```python
from build123d import *

# Parameters (mm, degrees)
CROQUIS1_W                   = 30
CROQUIS1_H                   = 10
CROQUIS1_R                   = 1.6
SALIENTE_EXTRUIR1_DEPTH      = 5
CROQUIS2_R                   = 2.8
CORTAR_EXTRUIR1_DEPTH        = 3
SALIENTE_EXTRUIR2_DEPTH      = 10
SALIENTE_EXTRUIR2_DEPTH_BACK = 30
CROQUIS3_W                   = 3
CROQUIS3_H                   = 40
CROQUIS4_W                   = 10
CROQUIS4_H                   = 5
SALIENTE_EXTRUIR3_DEPTH      = 10
SALIENTE_EXTRUIR4_DEPTH      = 10
REDONDEO1_R                  = 5


with BuildPart() as part:
    # Croquis1 → Saliente-Extruir1 (new body)
    with BuildSketch(Plane(origin=(0, 0, 0), x_dir=(1, 0, 0), z_dir=(0, 1, 0))):
        with Locations((15, 5)):
            Rectangle(CROQUIS1_W, CROQUIS1_H)
        with Locations(Location((5, 5, 0), (0, 0, 270))):
            Circle(CROQUIS1_R, mode=Mode.SUBTRACT)
        with Locations(Location((25, 5, 0), (0, 0, 270))):
            Circle(CROQUIS1_R, mode=Mode.SUBTRACT)
    extrude(amount=SALIENTE_EXTRUIR1_DEPTH)

    # Croquis2 → Cortar-Extruir1 (cut)
    with BuildSketch(Plane(origin=(0, 5, 0), x_dir=(1, 0, 0), z_dir=(0, 1, 0))):
        with Locations(Location((5, 5, 0), (0, 0, 270))):
            Circle(CROQUIS2_R)
        with Locations(Location((25, 5, 0), (0, 0, 270))):
            Circle(CROQUIS2_R)
    extrude(amount=-CORTAR_EXTRUIR1_DEPTH, mode=Mode.SUBTRACT)

    # Croquis3 → Saliente-Extruir2 (add, two sides: drawn at the far end of the back side and taken through both)
    with BuildSketch(Plane.ZY.offset(-SALIENTE_EXTRUIR2_DEPTH_BACK)):
        with Locations((-11.5, 20)):
            Rectangle(CROQUIS3_W, CROQUIS3_H)
    extrude(amount=SALIENTE_EXTRUIR2_DEPTH + SALIENTE_EXTRUIR2_DEPTH_BACK)

    # Croquis4 → Saliente-Extruir3 (add)
    with BuildSketch(Plane.ZY):
        with Locations((-5, 2.5)):
            Rectangle(CROQUIS4_W, CROQUIS4_H)
    extrude(amount=SALIENTE_EXTRUIR3_DEPTH)

    # Croquis5 → Saliente-Extruir4 (add)
    with BuildSketch(Plane(origin=(30, 0, 0), x_dir=(0, 0, -1), z_dir=(1, 0, 0))):
        Polygon((0, 0), (13, 0), (13, 40), (10, 40), (10, 5), (0, 5), align=None)
    extrude(amount=SALIENTE_EXTRUIR4_DEPTH)

    # Redondeo1
    # the kernel refuses this fillet: 5 mm, written as the material it adds along each edge
    with BuildSketch(Plane(origin=(40, 5, -10), x_dir=(0, 1, 0), z_dir=(-1, 0, 0))) as redondeo1_piece_1_section:
        with BuildLine():
            CenterArc((REDONDEO1_R, -REDONDEO1_R), REDONDEO1_R, 90, 90)
            Line((0, -REDONDEO1_R), (0, 0))
            Line((0, 0), (REDONDEO1_R, 0))
        make_face()
    redondeo1_piece_1 = extrude(amount=50, mode=Mode.PRIVATE)
    redondeo1_piece_1 = redondeo1_piece_1 - Plane(origin=(5, 6.156265405, -5), x_dir=(0, 0, 1), z_dir=(0, 1, 0)) * Cylinder(2.8, 120, mode=Mode.PRIVATE)
    redondeo1_piece_1 = redondeo1_piece_1 - Plane(origin=(25, 6.156265405, -5), x_dir=(0, 0, 1), z_dir=(0, 1, 0)) * Cylinder(2.8, 120, mode=Mode.PRIVATE)
    add(redondeo1_piece_1)


solid = part.part
```
Geometry: final body of the model. Coordinates: model frame, mm. A direction names the side the tool comes from. Coordinates: 2 decimals unless noted, no trailing zeros. Order: outer loops, then holes, each group sorted by start corner. A loop starts at its lowest first (then second) coordinate and runs counter-clockwise, first axis right, second up. Notation, with made-up numbers: (64.25, 8) - (101.25, 8) arc R28 cw to (101.25, 42) - close; hole circle Ø10 at (13.5, 86.25). An arc over 180 degrees is marked (long way). Return JSON: item names as keys, results as strings. Group by question number.
1. Set-up query: faces 1 (the face through (-10, 14.2, -10.4)), 2 (the face through (15, 5, -3)), 3 (the face through (5.1, 3.5, -7.8)). Return all of +Z, -Z, +X, -X, +Y, -Y with unobstructed straight access to the full face (end or side cutting, diameter ignored); none if empty.
2. Cut plane B-B (y = 3.5). Output: boundary loops of the cut face in (x, z).
3. Cut plane C-C (x = 12). Output: boundary loops of the cut face in (y, z).
4. Cut plane A-A (x = 5). Output: boundary loops of the cut face in (y, z).
5. Material intervals for line 1 along X through (y, z) = (4.95, -5); line 2 along X through (y, z) = (3, -6); line 3 along Z through (x, y) = (25, 4.75), sorted ascending. Write a range as [from, to].
6. Cut plane D-D (z = -1). Output: boundary loops of the cut face in (x, y), plus the area to 3 significant figures.
7. Pin query (flat end, axial travel): pin 1 (15 mm diameter, centred on x = 7.5, y = 30, fed in from +Z); pin 2 (7.5 mm diameter, centred on x = 5, z = -5, fed in from +Y); pin 3 (5.5 mm diameter, centred on x = 20.5, z = -3, fed in from +Y). Return the tip coordinate at first contact, or that it passes through.
8. Pull-direction query (X, two-part tool) for faces 4 (the face through (40, 14.2, -10.4)), 5 (the face through (24.03, 0.99, -6.27)), 6 (the face through (15, 40, -12)); classes: pulls with the +X half, pulls with the -X half, needs draft (parallel to the pull), parting line crosses it, or undercut.
Resolved:
{
 "1": {"face 1": "+Z, -Z, -X, +Y, -Y", "face 2": "+Z, +X, -X, +Y", "face 3": "+Y"},
 "2": {"outline": "(-10, -13) - (40, -13) - (40, 0) - (-10, 0) - close; hole circle Ø5.6 at (5, -5); hole circle Ø5.6 at (25, -5)"},
 "3": {"outline": "(0, -13) - (40, -13) - (40, -10) - (10, -10) arc R5 cw to (5, -5) - (5, 0) - (0, 0) - close"},
 "4": {"outline": "(0, -13) - (40, -13) - (40, -10) - (10, -10) arc R5 cw to (5.86, -7.8) - (2, -7.8) - (2, -6.6) - (0, -6.6) - close; (0, -3.4) - (2, -3.4) - (2, -2.2) - (5, -2.2) - (5, 0) - (0, 0) - close"},
 "5": {"line 1": "x = [-10, 2.2], [7.8, 22.2], [27.8, 40]", "line 2": "x = [-10, 2.38], [7.62, 22.38], [27.62, 40]", "line 3": "z = [-13, -7.8], [-2.2, 0]"},
 "6": {"outline": "(-10, 0) - (40, 0) - (40, 5) - (-10, 5) - close", "area": "250 mm²"},
 "7": {"pin 1": "stops at z = -10", "pin 2": "stops at y = 6.69", "pin 3": "stops at y = 5.06"},
 "8": {"face 4": "pulls with the +X half", "face 5": "undercut", "face 6": "needs draft"}
}
